```python
from build123d import *

# Parameters (mm, degrees)
CROQUIS1_R              = 1.5
SALIENTE_EXTRUIR1_DEPTH = 3


with BuildPart() as part:
    # Croquis1 → Saliente-Extruir1 (new body)
    with BuildSketch(Plane.XY):
        with BuildLine():
            Line((-27.735211809, 52.645866632), (-43.365211809, 52.645866632))
            Line((-43.365211809, 52.645866632), (-43.365211809, 55.645866632))
            Line((-43.365211809, 55.645866632), (-48.365211809, 55.645866632))
            Line((-48.365211809, 55.645866632), (-48.365211809, 52.645866632))
            Line((-48.365211809, 52.645866632), (-53.695211809, 52.645866632))
            ThreePointArc((-53.695211809, 52.645866632), (-56.523638933, 51.474293757), (-57.695211809, 48.645866632))
            Line((-57.695211809, 48.645866632), (-57.695211809, -16.854133368))
            ThreePointArc((-57.695211809, -16.854133368), (-56.523638933, -19.682560493), (-53.695211809, -20.854133368))
            Line((-53.695211809, -20.854133368), (-48.365211809, -20.854133368))
            Line((-48.365211809, -20.854133368), (-48.365211809, -23.854133368))
            Line((-48.365211809, -23.854133368), (-43.365211809, -23.854133368))
            Line((-43.365211809, -23.854133368), (-43.365211809, -20.854133368))
            Line((-43.365211809, -20.854133368), (-34.815211809, -20.854133368))
            Line((-34.815211809, -20.854133368), (-34.815211809, -23.854133368))
            Line((-34.815211809, -23.854133368), (-29.815211809, -23.854133368))
            Line((-29.815211809, -23.854133368), (-29.815211809, -20.854133368))
            Line((-29.815211809, -20.854133368), (-17.225211809, -20.854133368))
            ThreePointArc((-17.225211809, -20.854133368), (-14.396784684, -19.682560493), (-13.225211809, -16.854133368))
            Line((-13.225211809, -16.854133368), (-13.225211809, 48.645866632))
            ThreePointArc((-13.225211809, 48.645866632), (-14.396784684, 51.474293757), (-17.225211809, 52.645866632))
            Line((-17.225211809, 52.645866632), (-22.735211809, 52.645866632))
            Line((-22.735211809, 52.645866632), (-22.735211809, 55.645866632))
            Line((-22.735211809, 55.645866632), (-27.735211809, 55.645866632))
            Line((-27.735211809, 55.645866632), (-27.735211809, 52.645866632))
        make_face()
        with Locations((-55.195211809, 36.645866632)):
            Circle(CROQUIS1_R, mode=Mode.SUBTRACT)
        with Locations((-50.195211809, -15.354133368)):
            Circle(CROQUIS1_R, mode=Mode.SUBTRACT)
        with Locations((-22.195211809, -15.354133368)):
            Circle(CROQUIS1_R, mode=Mode.SUBTRACT)
        with BuildLine():
            Line((-35.550211809, 42.645866632), (-25.225211809, 42.645866632))
            ThreePointArc((-25.225211809, 42.645866632), (-23.810998246, 42.060080194), (-23.225211809, 40.645866632))
            Line((-23.225211809, 40.645866632), (-23.225211809, -8.854133368))
            ThreePointArc((-23.225211809, -8.854133368), (-23.810998246, -10.26834693), (-25.225211809, -10.854133368))
            Line((-25.225211809, -10.854133368), (-45.720101709, -10.854133368))
            ThreePointArc((-45.720101709, -10.854133368), (-47.125432715, -10.277174044), (-47.719944893, -8.879178133))
            Line((-47.719944893, -8.879178133), (-48.339851435, 40.620821867))
            ThreePointArc((-48.339851435, 40.620821867), (-47.763048927, 42.051197638), (-46.340008251, 42.645866632))
            Line((-46.340008251, 42.645866632), (-35.550211809, 42.645866632))
        make_face(mode=Mode.SUBTRACT)
    extrude(amount=SALIENTE_EXTRUIR1_DEPTH)


solid = part.part
```
Geometry check sheet. Reference: the model listing, model coordinates, mm. A direction names the side the tool comes from. Give positions to 0.01 mm unless a question says otherwise; leave off trailing zeros. Write each loop counter-clockwise with the first axis right and the second up, starting at its lowest first coordinate (ties: lowest second). Pieces come first, ordered by that corner, then holes. Notation, with made-up numbers: (-32, 34) -> (-20, 34) arc R13 ccw to (-20, 45) -> close; hole circle Ø1 at (22, -14.75). An arc over 180 degrees is marked (long way). One line per question, with ' | ' between items.
Item 1: Depth check by flat-ended pin: pin 1 (1 mm diameter, centred on x = -30.5, z = 1.5, fed in from +Y); pin 2 (1.5 mm diameter, centred on y = -22, z = 2, fed in from -X); pin 3 (1.8 mm diameter, centred on x = -55.2, y = 36.65, fed in from -Z). Enter the tip coordinate at first touch or a pass-through.
Determined:
pin 1: y = 52.65 | pin 2: x = -48.37 | pin 3: through
Item 2: Scan lines: line 1 along Y through (x, z) = (-33.5, 2.8); line 2 along X through (y, z) = (40, 0.5); line 3 along Y through (x, z) = (-43, 2). Record each from-to range of solid material in increasing order.
Determined:
line 1: -23.85 to -10.85, 42.65 to 52.65 | line 2: -57.7 to -48.33, -23.23 to -13.23 | line 3: -20.85 to -10.85, 42.65 to 52.65
Item 3: Sectioned sample at A-A, the plane x = -39. Record the boundary of the cut face in (y, z), plus the area to 3 significant figures.
Determined:
outline: (-20.85, 0) -> (-10.85, 0) -> (-10.85, 3) -> (-20.85, 3) -> close; (42.65, 0) -> (52.65, 0) -> (52.65, 3) -> (42.65, 3) -> close | area: 60.0 mm^2
Item 4: Sectioned sample at C-C, the plane x = -19.5. Record the boundary of the cut face in (y, z), plus the area to 4 significant figures.
Determined:
outline: (-20.85, 0) -> (52.65, 0) -> (52.65, 3) -> (-20.85, 3) -> close | area: 220.5 mm^2
Item 5: Draft check along X on faces 1 (the flat face through (-46, 55.646, 1)), 2 (the cylindrical face through (-48.8, -15.9, 1.5)), 3 (the flat face through (-13.225, 15, 1)). Enter one of: released by +X, released by -X, zero draft, split by the parting line, or undercut.
Determined:
face 1: zero draft | face 2: undercut | face 3: released by +X
Item 6: Sectioned sample at B-B, the plane y = 19. Record the boundary of the cut face in (x, z).
Determined:
outline: (-57.7, 0) -> (-48.07, 0) -> (-48.07, 3) -> (-57.7, 3) -> close; (-23.23, 0) -> (-13.23, 0) -> (-13.23, 3) -> (-23.23, 3) -> close
Item 7: Access from +Z, -Z, +X, -X, +Y, -Y to the whole of each face (thin tool, end or side, straight path). Record for faces 4 (the cylindrical face through (-23.83, 42.08, 1.48)), 5 (the flat face through (-27.735, 54, 1)), 6 (the flat face through (-43.365, -22, 1)), 7 (the flat face through (-20, 52.646, 1)).
Determined:
face 4: +Z, -Z | face 5: +Z, -Z, +Y | face 6: +Z, -Z, -Y | face 7: +Z, -Z, +X, +Y
Item 8: Sectioned sample at D-D, the plane z = 2.25. State how many separate pieces and enclosed holes the cut face has, plus the area to 3 significant figures.
Determined:
separate pieces: 1 | enclosed holes: 4 | area: 1,970 mm^2
